Geometry: final body of the model. Coordinates: model frame, mm. A direction names the side the tool comes from. Give positions to 0.01 mm unless a question says otherwise; leave off trailing zeros. Loops run counter-clockwise (first coordinate to the right, second up) from the corner with the lowest first, then second, coordinate; pieces in that order, holes last. Notation, with made-up numbers: (58.25, 22.25) - (63.25, 22.25) arc R9 ccw to (63.25, 36.25) - close; hole circle Ø3 at (57.5, -40). An arc over 180 degrees is marked (long way). Use one line per item in the form item = value.
```python
from build123d import *

# Parameters (mm, degrees)
SKETCH1_R             = 30
BOSS_EXTRUDE1_DEPTH   = 100
SKETCH2_R             = 30
SKETCH2_R_2           = 25
CUT_EXTRUDE1_DEPTH    = 40
BODY_MOVE_COPY1_ANGLE = 90


with BuildPart() as part:
    # Sketch1 → Boss-Extrude1 (new, symmetric)
    with BuildSketch(Plane.XY):
        Circle(SKETCH1_R)
    extrude(amount=BOSS_EXTRUDE1_DEPTH, both=True)

    # Sketch2 → Cut-Extrude1 (cut)
    with BuildSketch(Plane.XY.offset(100)):
        Circle(SKETCH2_R)
        Circle(SKETCH2_R_2, mode=Mode.SUBTRACT)
    cut_extrude1 = extrude(amount=-CUT_EXTRUDE1_DEPTH, mode=Mode.SUBTRACT)

    # Mirror1: Cut-Extrude1 across plane
    add(cut_extrude1.mirror(Plane.XY), mode=Mode.SUBTRACT)


with BuildPart() as body_2:
    # Body-Move/Copy1: copy of part
    add(part.part.rotate(Axis((0, 0, 0), (0, 1, 0)), BODY_MOVE_COPY1_ANGLE))


with BuildPart() as part_1:
    add(part.part)

    # Combine1: union body 2
    add(body_2.part)


solid = part_1.part
```
(1) Pin query (flat end, axial travel): P1, Ø6, axis at x = 46.5, y = 1.5, coming from the +Z side; P2, Ø5, axis at y = 2.5, z = -55.5, coming from the -X side; P3, Ø6, axis at x = -61, y = -19, coming from the -Z side. Return the tip coordinate at first contact, or that it passes through.
Solution:
P1 = 30
P2 = -30
P3 = -25.27
(2) Material intervals for L1, parallel to Z at x = -24, y = 10.5; L2, parallel to X at y = 27.5, z = -24, sorted ascending. Write a range as from..to.
Solution:
L1 = -60..60
L2 = -11.99..11.99
(3) Cut plane A-A (y = 0). Return the cut outline in (x, z).
Solution:
outline = (-100, -25) - (-60, -25) - (-60, -30) - (-30, -30) - (-30, -60) - (-25, -60) - (-25, -100) - (25, -100) - (25, -60) - (30, -60) - (30, -30) - (60, -30) - (60, -25) - (100, -25) - (100, 25) - (60, 25) - (60, 30) - (30, 30) - (30, 60) - (25, 60) - (25, 100) - (-25, 100) - (-25, 60) - (-30, 60) - (-30, 30) - (-60, 30) - (-60, 25) - (-100, 25) - close
(4) Access query for faces 1 (the face through (23.846, 7.509, 80.28)), 2 (the face through (80.28, 7.509, -23.846)), 3 (the face through (23.846, 7.509, -80.28)), 4 (the face through (-36.247, 9.011, -28.615)). Directions: +Z, -Z, +X, -X, +Y, -Y. A direction counts if a zero-diameter tool reaches every point of the face in a straight line with its end or side. Return the directions, or none.
Solution:
face_1 = +Z
face_2 = +X
face_3 = -Z
face_4 = -X
(5) Cut plane D-D (y = -20.5). Return the cut outline in (x, z), plus the area to 3 significant figures.
Solution:
outline = (-100, -14.31) - (-60, -14.31) - (-60, -21.9) - (-21.9, -21.9) - (-21.9, -60) - (-14.31, -60) - (-14.31, -100) - (14.31, -100) - (14.31, -60) - (21.9, -60) - (21.9, -21.9) - (60, -21.9) - (60, -14.31) - (100, -14.31) - (100, 14.31) - (60, 14.31) - (60, 21.9) - (21.9, 21.9) - (21.9, 60) - (14.31, 60) - (14.31, 100) - (-14.31, 100) - (-14.31, 60) - (-21.9, 60) - (-21.9, 21.9) - (-60, 21.9) - (-60, 14.31) - (-100, 14.31) - close
area = 13,200 mm2
(6) Cut plane B-B (x = -16). Return the cut outline in (y, z).
Solution:
outline = (-25.38, -60) - (-19.21, -60) - (-19.21, -100) - (19.21, -100) - (19.21, -60) - (25.38, -60) - (25.38, -16) arc R30 ccw to (25.38, 16) - (25.38, 60) - (19.21, 60) - (19.21, 100) - (-19.21, 100) - (-19.21, 60) - (-25.38, 60) - (-25.38, 16) arc R30 ccw to (-25.38, -16) - close
(7) Cut plane C-C (z = -50.5). Return the cut outline in (x, y), plus the area to 3 significant figures.
Solution:
outline = circle Ø60 at (0, 0)
area = 2,830 mm2
